```python
from build123d import *

# Parameters (mm, degrees)
F1_DEPTH = 25


with BuildPart() as f1:
    # F0 (on Top) → F1 (new body)
    with BuildSketch(Plane.XY):
        Polygon((-54.724703, 0), (-54.724703, -30), (45.275297, -30), (45.275297, 0), (20.275297, 0), (20.275297, -18.218007), (-29.724703, -18.218007), (-29.724703, 0), align=None)
        Polygon((-34.724703, 16.781993), (-54.724703, 0), (-29.724703, 0), (-29.724703, 1.781993), (-14.724703, 1.781993), (-14.724703, 16.781993), align=None)
        Polygon((20.275297, 0), (45.275297, 0), (25.275297, 16.781993), (5.275297, 16.781993), (5.275297, 1.781993), (20.275297, 1.781993), align=None)
    extrude(amount=F1_DEPTH)


solid = f1.part
```
CAD build for the part. Positions are in the model's coordinates, mm. A direction names the side the tool comes from. Round coordinates to 2 decimals unless told otherwise and drop trailing zeros. Order: outer loops, then holes, each group sorted by start corner. A loop starts at its lowest first (then second) coordinate and runs counter-clockwise, first axis right, second up.
Item 1: Saw through at D-D on x = -1. Write the cut outline in (y, z).
Item 2: Mould opens along X. For faces 1 (the face through (35.42, 8.27, 12.32)), 2 (the face through (-25, 16.782, 12)), 3 (the face through (-22, 1.782, 12)) say: pulls with the +X half, pulls with the -X half, needs draft (parallel to the pull), parting line crosses it, or undercut.
Item 3: Tool access for faces 4 (the face through (5.275, 9, 12)), 5 (the face through (-5, -22, 0)), 6 (the face through (-29.725, -8, 12)): list every direction of +Z, -Z, +X, -X, +Y, -Y with a clear straight run to the whole face (end or side of a thin tool).
Item 4: Saw through at C-C on z = 3. Write the cut outline in (x, y), then the cut area to 3 significant figures.
Item 5: Saw through at B-B on x = -27. Write the cut outline in (y, z), then the cut area to 3 significant figures.
Item 6: Pin check, flat tips, straight feed: pin 1 (8 mm diameter, centred on x = -42.5, z = 8, fed in from +Y); pin 2 (7.5 mm diameter, centred on y = 6, z = 15, fed in from -X). Stop position of each tip, or through.
Item 7: Probe line 1 along X through (y, z) = (-10.5, 13); line 2 along Y through (x, z) = (-19.5, 21.5); line 3 along Y through (x, z) = (2, 6.25). List the from-to ranges inside material, lowest first.
Item 8: Saw through at A-A on y = -3. Write the cut outline in (x, z), then the cut area to 3 significant figures.
Reported:
1. outline: (-30, 0) - (-18.22, 0) - (-18.22, 25) - (-30, 25) - close
2. face 1: pulls with the +X half
2. face 2: needs draft
2. face 3: undercut
3. face 4: +Z, -Z, +Y
3. face 5: -Z, +X, -X, +Y, -Y
3. face 6: +Z, -Z
4. outline: (-54.72, -30) - (45.28, -30) - (45.28, 0) - (25.28, 16.78) - (5.28, 16.78) - (5.28, 1.78) - (20.28, 1.78) - (20.28, -18.22) - (-29.72, -18.22) - (-29.72, 1.78) - (-14.72, 1.78) - (-14.72, 16.78) - (-34.72, 16.78) - (-54.72, 0) - close
4. area: 3,040 mm2
5. outline: (-30, 0) - (-18.22, 0) - (-18.22, 25) - (-30, 25) - close; (1.78, 0) - (16.78, 0) - (16.78, 25) - (1.78, 25) - close
5. area: 670 mm2
6. pin 1: stops at y = 13.61
6. pin 2: stops at x = -52.04
7. line 1: x = -54.72 to -29.72, 20.28 to 45.28
7. line 2: y = -30 to -18.22, 1.78 to 16.78
7. line 3: y = -30 to -18.22
8. outline: (-54.72, 0) - (-29.72, 0) - (-29.72, 25) - (-54.72, 25) - close; (20.28, 0) - (45.28, 0) - (45.28, 25) - (20.28, 25) - close
8. area: 1,250 mm2
